from build123d import *

# Parameters (mm, degrees)
SKETCH_1_W          = 6
SKETCH_1_H          = 6
SKETCH_1_R          = 1.5
EXTRUDE_1_DEPTH     = 6
SKETCH_2_R          = 1.5
CUT_EXTRUDE_1_DEPTH = 6
SKETCH_3_R          = 1.5
CUT_EXTRUDE_2_DEPTH = 6


with BuildPart() as part:
    # 草图1 → 凸台-拉伸1 (new body)
    with BuildSketch(Plane(origin=(0, 0, 0), x_dir=(1, 0, 0), z_dir=(0, 1, 0))):
        with Locations((3, 3)):
            Rectangle(SKETCH_1_W, SKETCH_1_H)
        with Locations(Location((3, 3, 0), (0, 0, 270))):
            Circle(SKETCH_1_R, mode=Mode.SUBTRACT)
    extrude(amount=EXTRUDE_1_DEPTH)

    # 草图2 → 切除-拉伸1 (cut)
    with BuildSketch(Plane.XY):
        with Locations((3, 3)):
            Circle(SKETCH_2_R)
    extrude(amount=-CUT_EXTRUDE_1_DEPTH, mode=Mode.SUBTRACT)

    # 草图3 → 切除-拉伸2 (cut)
    with BuildSketch(Plane(origin=(6, 0, 0), x_dir=(0, 0, -1), z_dir=(1, 0, 0))):
        with Locations((3, 3)):
            Circle(SKETCH_3_R)
    extrude(amount=-CUT_EXTRUDE_2_DEPTH, mode=Mode.SUBTRACT)


solid = part.part
For this review, take the finished solid that the model builds, in its own axes (mm). Coordinates: 2 decimals unless noted, no trailing zeros. Order: outer loops, then holes, each group sorted by start corner. A loop starts at its lowest first (then second) coordinate and runs counter-clockwise, first axis right, second up. Notation, with made-up numbers: (-38, 52) - (10, 52) arc R27 ccw to (10, 75) - close; hole circle Ø3 at (75.5, 51). An arc over 180 degrees is marked (long way). Answer as CSV lines item,"result". Start each with the question number.
1) Add section A-A (y = 3). State the section outline as (x, z) points, then the cut area to 3 significant figures.
2) Insertion check: P1, Ø1.8, axis at x = 3, y = 3, coming from the +Z side. The pin has a flat end and moves straight along its axis. Give the tip position at first contact, or say it passes through.
3) To check wall thickness, follow line 1 along Y through (x, z) = (3, -4.85); line 2 along Z through (x, y) = (3, 0.9). State the ranges of each line that lie inside material, in increasing order. Write a range as [from, to].
4) Draft analysis for pull direction X (two halves, no side actions). For faces 1 (the flat face through (1.6, 6, -4.4)), 2 (the cylindrical face through (1.89, 4.01, -5.23)), 3 (the flat face through (0, 1.6, -1.6)), state which applies: +X half, -X half, draft (parallel to the pull), parting line (faces both ways), or undercut.
5) Add section C-C (x = 4.8). State the section outline as (y, z) points.
6) Add section D-D (z = -5.15). State the section outline as (x, y) points, then the cut area to 3 significant figures.
Result:
1,outline,"(0, -6) - (1.5, -6) - (1.5, -4.5) - (0, -4.5) - close; (0, -1.5) - (1.5, -1.5) - (1.5, 0) - (0, 0) - close; (4.5, -6) - (6, -6) - (6, -4.5) - (4.5, -4.5) - close; (4.5, -1.5) - (6, -1.5) - (6, 0) - (4.5, 0) - close"
1,area,"9.00 mm^2"
2,P1,"through"
3,line 1,"[0, 1.5], [4.5, 6]"
3,line 2,"[-6, -4.5], [-1.5, 0]"
4,face 1,"draft"
4,face 2,"undercut"
4,face 3,"-X half"
5,outline,"(0, -6) - (6, -6) - (6, 0) - (0, 0) - close; hole circle Ø3 at (3, -3)"
6,outline,"(0, 0) - (6, 0) - (6, 6) - (0, 6) - close; hole circle Ø3 at (3, 3)"
6,area,"28.9 mm^2"
